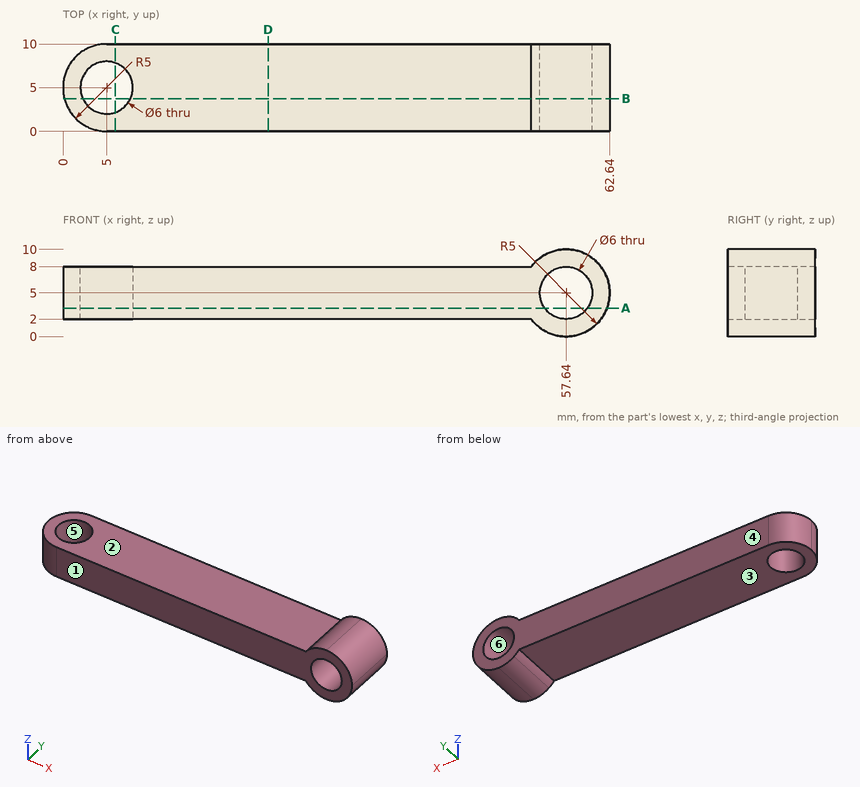
For this review, use the dimensioned drawing (mm, ordinates from the lowest corner) and the shaded views. A direction names the side the tool comes from. Round coordinates to 2 decimals unless told otherwise and drop trailing zeros. Write each loop counter-clockwise with the first axis right and the second up, starting at its lowest first coordinate (ties: lowest second). Pieces come first, ordered by that corner, then holes. Notation, with made-up numbers: (-15.5, -17.5) - (-5.5, -17.5) arc R15 cw to (-5.5, 1.5) - close; hole circle Ø1 at (-22, 77). An arc over 180 degrees is marked (long way). Answer as CSV lines item,"result". Start each with the question number.
(1) To check wall thickness, follow line 1 (Y direction, x = 5, z = 4.15); line 2 (X direction, y = 4.5, z = 5.75); line 3 (X direction, y = 4, z = 3.75). State the ranges of each line that lie inside material, in increasing order.
(2) We need section B-B on y = 3.75. State the section outline as (x, z) points.
(3) For pin 1 Ø2 at (x, y) = (13, 3) entering from +Z; pin 2 Ø2 at (x, y) = (49, 1.5) entering from -Z; pin 3 Ø3.5 at (x, y) = (5, 5) entering from -Z; pin 4 Ø4 at (y, z) = (6.5, 7.5) entering from +X, all flat-tipped, find the tip position at first contact; note any pin that passes through.
(4) We need section D-D on x = 23.5. State the section outline as (y, z) points.
(5) For the marked faces 1, 2 and 3, list the 3-axis set-ups (+Z, -Z, +X, -X, +Y, -Y) from which the entire face can be reached by the end or side of a thin tool; tool diameter is ignored.
(6) We need section A-A on z = 3.25. State the section outline as (x, y) points, plus the area to 4 significant figures.
(7) Draft analysis for pull direction X (two halves, no side actions). For the marked faces 4, 5 and 6, state which applies: pulls with the +X half, pulls with the -X half, needs draft (parallel to the pull), parting line crosses it, or undercut.
(8) We need section C-C on x = 6. State the section outline as (y, z) points.
Worked answers:
1,line 1,"0 to 2, 8 to 10"
1,line 2,"0.03 to 2.04, 7.96 to 54.74, 60.54 to 62.58"
1,line 3,"0.1 to 2.17, 7.83 to 54.91, 60.37 to 62.48"
2,outline,"(0.16, 2) - (2.27, 2) - (2.27, 8) - (0.16, 8) - close; (7.73, 2) - (53.64, 2) arc R5 ccw (long way) to (53.64, 8) - (7.73, 8) - close; hole circle Ø6 at (57.64, 5)"
3,pin 1,"z = 8"
3,pin 2,"z = 2"
3,pin 3,"through"
3,pin 4,"x = 62.61"
4,outline,"(0, 2) - (10, 2) - (10, 8) - (0, 8) - close"
5,face 1,"+Z, -Z, +X, -X, -Y"
5,face 2,"+Z, -X, +Y, -Y"
5,face 3,"-Z, -X, +Y, -Y"
6,outline,"(5, 0) - (55.2, 0) - (55.2, 10) - (5, 10) arc R5 ccw to start; (60.08, 0) - (62.32, 0) - (62.32, 10) - (60.08, 10) - close; hole circle Ø6 at (5, 5)"
6,area,"535.5 mm²"
7,face 4,"needs draft"
7,face 5,"undercut"
7,face 6,"undercut"
8,outline,"(0, 2) - (2.17, 2) - (2.17, 8) - (0, 8) - close; (7.83, 2) - (10, 2) - (10, 8) - (7.83, 8) - close"
